Build history of the part. All positions in model axes, mm. Face numbers are marked on the shaded views. Round coordinates to 2 decimals unless told otherwise and drop trailing zeros. Write each loop counter-clockwise with the first axis right and the second up, starting at its lowest first coordinate (ties: lowest second). Pieces come first, ordered by that corner, then holes. Notation, with made-up numbers: M -23.75,72 L 3.25,72 A24 cw 3.25,84 Z; hole C 71,27 d5. An arc over 180 degrees is marked long. Write item = value, one per line. Start each with the question number.
Q1. Band-saw the part on C-C on z = 16. Write the cut outline in (x, y), plus the area to 3 significant figures.
Q2. Band-saw the part on D-D on z = 21.5. Write the cut outline in (x, y) (3 decimals), plus the area to 3 significant figures.
Q3. Pull direction Y, two halves, no side cores. Call the marked faces 1, 2 and 3: released by +Y, released by -Y, zero draft, split by the parting line, or undercut.
Q4. Probe L1, parallel to Y at x = 0, z = 18; L2, parallel to Z at x = 5.25, y = 2.25; L3, parallel to Y at x = 2, z = 9.75. List the from-to ranges inside material, lowest first.
Q5. Band-saw the part on A-A on y = 0. Write the cut outline in (x, z).
Q6. Drop flat-ended pins along their axis: P1, Ø10, axis at x = 10, z = 13.5, coming from the -Y side; P2, Ø1.5, axis at x = -0.5, z = 5.5, coming from the +Y side; P3, Ø4, axis at x = -5.5, z = 17.5, coming from the +Y side; P4, Ø1, axis at x = -2, z = 17.5, coming from the -Y side. Give the stop position or say it passes through.
```python
from build123d import *

# Parameters (mm, degrees)
F0_R     = 4.5
F1_DEPTH = 25
F0_R_2   = 12.75
F2_DEPTH = 2
F3_SIZE2 = 6
F3_SIZE  = 1.5
F4_D     = 5
F5_SIZE2 = 1
F5_SIZE  = 1


with BuildPart() as f1:
    # F0 (on Top) → F1 (new body)
    with BuildSketch(Plane.XY):
        Circle(F0_R)
    extrude(amount=F1_DEPTH)

    # F0 (on Top) → F2 (join)
    with BuildSketch(Plane.XY):
        Circle(F0_R_2)
        Circle(F0_R, mode=Mode.SUBTRACT)
    extrude(amount=F2_DEPTH)

    # F3
    f3_edges = [f1.edges().sort_by_distance(p)[0] for p in [
        (-4.5, 0, 25),
    ]]
    f3_side = f1.faces().sort_by_distance((0, 0, 25))[0]
    chamfer(f3_edges, length=F3_SIZE, length2=F3_SIZE2, reference=f3_side)

    # F4 (through all)
    with Locations(Plane(origin=(0, 0, 0), x_dir=(1, 0, 0), z_dir=(0, 0, -1))):
        with Locations((0, 0)):
            Hole(F4_D / 2)

    # F5
    f5_edges = [f1.edges().sort_by_distance(p)[0] for p in [
        (-12.75, 0, 2),
    ]]
    chamfer(f5_edges, length=F5_SIZE, length2=F5_SIZE2)


solid = f1.part
```
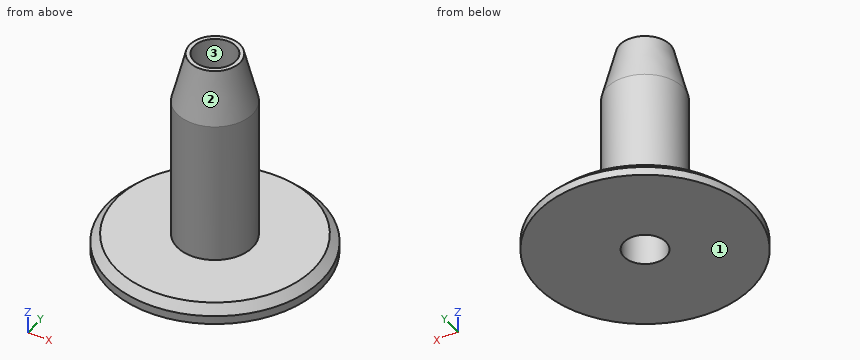
Conclusion:
q1.outline = C 0,0 d9; hole C 0,0 d5
q1.area = 44.0 mm^2
q2.outline = C 0,0 d7.75; hole C 0,0 d5
q2.area = 27.5 mm^2
q3.face_1 = zero draft
q3.face_2 = split by the parting line
q3.face_3 = undercut
q4.L1 = -4.5 to -2.5, 2.5 to 4.5
q4.L2 = 0 to 2
q4.L3 = -4.03 to -1.5, 1.5 to 4.03
q5.outline = M -12.75,0 L -2.5,0 L -2.5,25 L -3,25 L -4.5,19 L -4.5,2 L -11.75,2 L -12.75,1 Z; M 2.5,0 L 12.75,0 L 12.75,1 L 11.75,2 L 4.5,2 L 4.5,19 L 3,25 L 2.5,25 Z
q6.P1 = through
q6.P2 = 4.5
q6.P3 = 2.83
q6.P4 = -4.24
